```python
from build123d import *

# Parameters (mm, degrees)
F1_DEPTH = 25.4
F2_W     = 25.4
F2_H     = 25.4
F3_DEPTH = 25.4


with BuildPart() as f1:
    # F0 (on Front) → F1 (new body)
    with BuildSketch(Plane.XZ):
        with BuildLine():
            Line((-372.618, 12.7), (-347.218, 12.7))
            Line((-347.218, 12.7), (-347.218, -12.7))
            Line((-347.218, -12.7), (-372.618, -12.7))
            ThreePointArc((-372.618, -12.7), (-361.458768, -39.640768), (-334.518, -50.8))
            Line((-334.518, -50.8), (0, -50.8))
            Line((0, -50.8), (334.518, -50.8))
            ThreePointArc((334.518, -50.8), (361.458768, -39.640768), (372.618, -12.7))
            Line((372.618, -12.7), (347.218, -12.7))
            Line((347.218, -12.7), (347.218, 12.7))
            Line((347.218, 12.7), (372.618, 12.7))
            ThreePointArc((372.618, 12.7), (361.458768, 39.640768), (334.518, 50.8))
            Line((334.518, 50.8), (0, 50.8))
            Line((0, 50.8), (-334.518, 50.8))
            ThreePointArc((-334.518, 50.8), (-361.458768, 39.640768), (-372.618, 12.7))
        make_face()
        with BuildLine():
            Line((-38.1, -25.4), (-309.118, -25.4))
            ThreePointArc((-309.118, -25.4), (-318.098256, -21.680256), (-321.818, -12.7))
            Line((-321.818, -12.7), (-321.818, 12.7))
            ThreePointArc((-321.818, 12.7), (-318.098256, 21.680256), (-309.118, 25.4))
            Line((-309.118, 25.4), (-38.1, 25.4))
            ThreePointArc((-38.1, 25.4), (-29.119744, 21.680256), (-25.4, 12.7))
            Line((-25.4, 12.7), (-25.4, -12.7))
            ThreePointArc((-25.4, -12.7), (-29.119744, -21.680256), (-38.1, -25.4))
        make_face(mode=Mode.SUBTRACT)
        with BuildLine():
            Line((321.818, 12.7), (321.818, -12.7))
            ThreePointArc((321.818, -12.7), (318.098256, -21.680256), (309.118, -25.4))
            Line((309.118, -25.4), (38.1, -25.4))
            ThreePointArc((38.1, -25.4), (29.119744, -21.680256), (25.4, -12.7))
            Line((25.4, -12.7), (25.4, 12.7))
            ThreePointArc((25.4, 12.7), (29.119744, 21.680256), (38.1, 25.4))
            Line((38.1, 25.4), (309.118, 25.4))
            ThreePointArc((309.118, 25.4), (318.098256, 21.680256), (321.818, 12.7))
        make_face(mode=Mode.SUBTRACT)
    extrude(amount=F1_DEPTH)

    # F2 (on face) → F3 (cut)
    with BuildSketch(Plane.XZ.offset(25.4)):
        with Locations((0, 38.1)):
            Rectangle(F2_W, F2_H)
        with Locations((0, -38.1)):
            Rectangle(F2_W, F2_H)
    extrude(amount=-F3_DEPTH, mode=Mode.SUBTRACT)


solid = f1.part
```
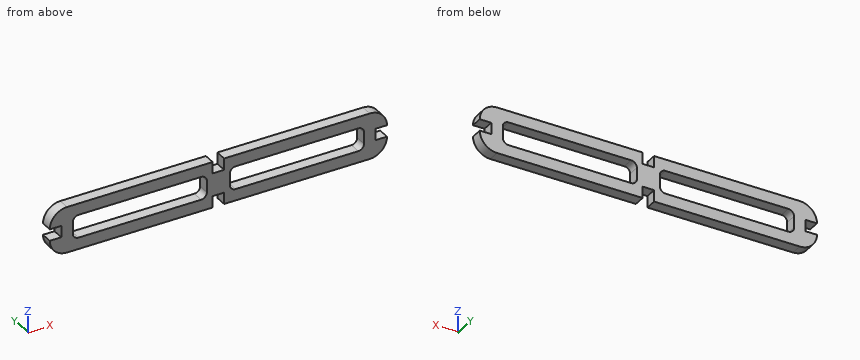
Part model, mm, in its own coordinate system. Round coordinates to 2 decimals unless told otherwise and drop trailing zeros. Loops run counter-clockwise (first coordinate to the right, second up) from the corner with the lowest first, then second, coordinate; pieces in that order, holes last.
1. Slice it at C-C (z = 40). Give the cut face in (x, y).
Solutions:
outline: (-361.09, -25.4) - (-12.7, -25.4) - (-12.7, 0) - (-361.09, 0) - close; (12.7, -25.4) - (361.09, -25.4) - (361.09, 0) - (12.7, 0) - close
2. Flat gauge pins, fed straight in: pin 1 (12.5 mm diameter, centred on y = -15, z = -5.5, fed in from -X); pin 2 (12.5 mm diameter, centred on y = -14, z = 0.5, fed in from +X); pin 3 (7.5 mm diameter, centred on x = -356.5, y = -18.5, fed in from +Z); pin 4 (12 mm diameter, centred on y = -5, z = -16, fed in from -X). Where does each tip first touch, or does it go through?
Solutions:
pin 1: stops at x = -347.22
pin 2: stops at x = 347.22
pin 3: stops at z = 46.15
pin 4: stops at x = -372.62
3. Drill centre lines: line 1 along X through (y, z) = (-19, 6); line 2 along Z through (x, y) = (-63, -9); line 3 along X through (y, z) = (-5.75, 23.5). Where is each one in solid material? Low to high.
Solutions:
line 1: x = -347.22 to -321.82, -25.4 to 25.4, 321.82 to 347.22
line 2: z = -50.8 to -25.4, 25.4 to 50.8
line 3: x = -371.06 to -315.8, -31.42 to 31.42, 315.8 to 371.06
4. Slice it at B-B (x = -203.5). Give the cut face in (y, z), and give its area (3 significant figures).
Solutions:
outline: (-25.4, -50.8) - (0, -50.8) - (0, -25.4) - (-25.4, -25.4) - close; (-25.4, 25.4) - (0, 25.4) - (0, 50.8) - (-25.4, 50.8) - close
area: 1,290 mm2
5. Slice it at D-D (y = -8.25). Count the separate pieces of the cut face and the enclosed holes in it, and give its area (4 significant figures).
Solutions:
separate pieces: 1
enclosed holes: 2
area: 42,050 mm2
6. Slice it at A-A (z = 3.5). Give the cut face in (x, y), and give its area (3 significant figures).
Solutions:
outline: (-347.22, -25.4) - (-321.82, -25.4) - (-321.82, 0) - (-347.22, 0) - close; (-25.4, -25.4) - (25.4, -25.4) - (25.4, 0) - (-25.4, 0) - close; (321.82, -25.4) - (347.22, -25.4) - (347.22, 0) - (321.82, 0) - close
area: 2,580 mm2
